from build123d import *

# Parameters (mm, degrees)
SKETCH1_R      = 2.5
SKETCH1_R_2    = 1
EXTRUDE1_DEPTH = 2
FILLET1_R      = 1


with BuildPart() as part:
    # Sketch1 → Extrude1 (new body)
    with BuildSketch(Plane.XY):
        with BuildLine():
            Line((3, 13.5), (3, 5.196152423))
            Line((3, 5.196152423), (10.191342951, 9.348076211))
            ThreePointArc((10.191342951, 9.348076211), (14.289419162, 8.25), (13.191342951, 4.151923789))
            Line((13.191342951, 4.151923789), (6, 0))
            Line((6, 0), (13.191342951, -4.151923789))
            ThreePointArc((13.191342951, -4.151923789), (14.289419162, -8.25), (10.191342951, -9.348076211))
            Line((10.191342951, -9.348076211), (3, -5.196152423))
            Line((3, -5.196152423), (3, -13.5))
            ThreePointArc((3, -13.5), (0, -16.5), (-3, -13.5))
            Line((-3, -13.5), (-3, -5.196152423))
            Line((-3, -5.196152423), (-10.191342951, -9.348076211))
            ThreePointArc((-10.191342951, -9.348076211), (-14.289419162, -8.25), (-13.191342951, -4.151923789))
            Line((-13.191342951, -4.151923789), (-6, 0))
            Line((-6, 0), (-13.191342951, 4.151923789))
            ThreePointArc((-13.191342951, 4.151923789), (-14.289419162, 8.25), (-10.191342951, 9.348076211))
            Line((-10.191342951, 9.348076211), (-3, 5.196152423))
            Line((-3, 5.196152423), (-3, 13.5))
            ThreePointArc((-3, 13.5), (0, 16.5), (3, 13.5))
        make_face()
        Circle(SKETCH1_R, mode=Mode.SUBTRACT)
        with Locations((0, 7.5)):
            Circle(SKETCH1_R_2, mode=Mode.SUBTRACT)
        with Locations((0, 10.5)):
            Circle(SKETCH1_R_2, mode=Mode.SUBTRACT)
        with Locations((0, 13.5)):
            Circle(SKETCH1_R_2, mode=Mode.SUBTRACT)
        with Locations((-6.495190528, 3.75)):
            Circle(SKETCH1_R_2, mode=Mode.SUBTRACT)
        with Locations((-9.09326674, 5.25)):
            Circle(SKETCH1_R_2, mode=Mode.SUBTRACT)
        with Locations((-11.691342951, 6.75)):
            Circle(SKETCH1_R_2, mode=Mode.SUBTRACT)
        with Locations((-6.495190528, -3.75)):
            Circle(SKETCH1_R_2, mode=Mode.SUBTRACT)
        with Locations((-9.09326674, -5.25)):
            Circle(SKETCH1_R_2, mode=Mode.SUBTRACT)
        with Locations((-11.691342951, -6.75)):
            Circle(SKETCH1_R_2, mode=Mode.SUBTRACT)
        with Locations((0, -7.5)):
            Circle(SKETCH1_R_2, mode=Mode.SUBTRACT)
        with Locations((0, -10.5)):
            Circle(SKETCH1_R_2, mode=Mode.SUBTRACT)
        with Locations((0, -13.5)):
            Circle(SKETCH1_R_2, mode=Mode.SUBTRACT)
        with Locations((6.495190528, -3.75)):
            Circle(SKETCH1_R_2, mode=Mode.SUBTRACT)
        with Locations((9.09326674, -5.25)):
            Circle(SKETCH1_R_2, mode=Mode.SUBTRACT)
        with Locations((11.691342951, -6.75)):
            Circle(SKETCH1_R_2, mode=Mode.SUBTRACT)
        with Locations((6.495190528, 3.75)):
            Circle(SKETCH1_R_2, mode=Mode.SUBTRACT)
        with Locations((9.09326674, 5.25)):
            Circle(SKETCH1_R_2, mode=Mode.SUBTRACT)
        with Locations((11.691342951, 6.75)):
            Circle(SKETCH1_R_2, mode=Mode.SUBTRACT)
    extrude(amount=EXTRUDE1_DEPTH)

    # Fillet1
    fillet1_edges = [part.edges().sort_by_distance(p)[0] for p in [
        (3, 5.196152423, 1),
        (6, 0, 1),
        (3, -5.196152423, 1),
        (-3, -5.196152423, 1),
        (-6, 0, 1),
        (-3, 5.196152423, 1),
    ]]
    fillet(fillet1_edges, radius=FILLET1_R)


solid = part.part
Build history of the part. All positions in model axes, mm. A direction names the side the tool comes from. Coordinates: 2 decimals unless noted, no trailing zeros. Write each loop counter-clockwise with the first axis right and the second up, starting at its lowest first coordinate (ties: lowest second). Pieces come first, ordered by that corner, then holes. Notation, with made-up numbers: (73.5, 13) -> (79.5, 13) arc R21 cw to (79.5, 25) -> close; hole circle Ø9 at (40, 0.5). An arc over 180 degrees is marked (long way). Use CSV: the item, a comma, the result in double quotes. Start each with the question number.
Q1. Pull direction X, two halves, no side cores. Call faces 4 (the cylindrical face through (0.1, -16.5, 1)), 5 (the cylindrical face through (-0.13, 8.49, 0.99)), 6 (the flat face through (10.31, -2.49, 0.99)): released by +X, released by -X, zero draft, split by the parting line, or undercut.
Q2. Flat gauge pins, fed straight in: pin 1 Ø3 at (x, y) = (0, 0) entering from -Z; pin 2 Ø0.6 at (y, z) = (-10.5, 1) entering from +X; pin 3 Ø1 at (y, z) = (9, 2) entering from +X. Where does each tip first touch, or does it go through?
Q3. Drill centre lines: probe 1 along Y at (x, z) = (-8.75, 1.75); probe 2 along X at (y, z) = (-13, 1.1); probe 3 along Y at (x, z) = (9.5, 1.5). Where is each one in solid material? Low to high.
Q4. Cut at D-D, the plane z = 0.7. State how many separate pieces and enclosed holes the cut face has, then the cut area to 3 significant figures.
Q5. 3-axis set-ups, long thin cutter, end or side, ignore diameter. For faces 1 (the flat face through (7.39, -7.73, 0.99)), 2 (the flat face through (-7.39, 7.73, 0.99)), 3 (the cylindrical face through (8.36, 5.93, 0.99)): which of +Z, -Z, +X, -X, +Y, -Y reach the whole face in a straight line?
Q6. Cut at A-A, the plane y = -10.5. List the corners of the cut face in (x, z), then the cut area to 3 significant figures.
Q7. Cut at C-C, the plane y = 5.25. List the corners of the cut face in (x, z), then the cut area to 3 significant figures.
Q8. Cut at B-B, the plane x = 11.75. List the corners of the cut face in (y, z).
Checked values:
1,face 4,"split by the parting line"
1,face 5,"undercut"
1,face 6,"released by +X"
2,pin 1,"passes through"
2,pin 2,"stops at x = 3"
2,pin 3,"stops at x = 14.13"
3,probe 1,"y = -8.52 to -6.19, -4.31 to -1.59, 1.59 to 4.31, 6.19 to 8.52"
3,probe 2,"x = -3 to -0.87, 0.87 to 3"
3,probe 3,"y = -8.95 to -6.16, -4.34 to -2.02, 2.02 to 4.34, 6.16 to 8.95"
4,separate pieces,"1"
4,enclosed holes,"19"
4,area,"405 mm²"
5,face 1,"+Z, -Z, -Y"
5,face 2,"+Z, -Z, +Y"
5,face 3,"+Z, -Z"
6,outline,"(-3, 0) -> (-1, 0) -> (-1, 2) -> (-3, 2) -> close; (1, 0) -> (3, 0) -> (3, 2) -> (1, 2) -> close"
6,area,"8.00 mm²"
7,outline,"(-14.29, 0) -> (-10.09, 0) -> (-10.09, 2) -> (-14.29, 2) -> close; (-8.09, 0) -> (8.09, 0) -> (8.09, 2) -> (-8.09, 2) -> close; (10.09, 0) -> (14.29, 0) -> (14.29, 2) -> (10.09, 2) -> close"
7,area,"49.2 mm²"
8,outline,"(-9.75, 0) -> (-7.75, 0) -> (-7.75, 2) -> (-9.75, 2) -> close; (-5.75, 0) -> (-3.32, 0) -> (-3.32, 2) -> (-5.75, 2) -> close; (3.32, 0) -> (5.75, 0) -> (5.75, 2) -> (3.32, 2) -> close; (7.75, 0) -> (9.75, 0) -> (9.75, 2) -> (7.75, 2) -> close"
